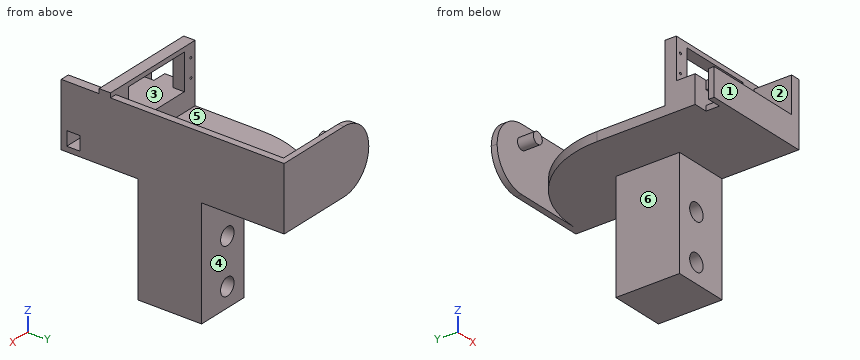
```python
from build123d import *

# Parameters (mm, degrees)
SKETCH1_W            = 55.49400001
SKETCH1_H            = 26.874
BOSS_EXTRUDE1_DEPTH  = 6.35
SKETCH2_W            = 40
SKETCH2_H            = 19
CUT_EXTRUDE1_DEPTH   = 6.35
SKETCH3_R            = 0.635
CUT_EXTRUDE2_DEPTH   = 6.35
SKETCH4_W            = 55.49400001
SKETCH4_H            = 7.874
BOSS_EXTRUDE2_DEPTH  = 21.15
SKETCH6_W            = 7.747000005
SKETCH6_H            = 6.35
BOSS_EXTRUDE3_DEPTH  = 1
SKETCH12_W           = 7.747000005
SKETCH12_H           = 7.475
CUT_EXTRUDE4_DEPTH   = 9.398
SKETCH13_W           = 7.747000005
SKETCH13_H           = 7.9
BOSS_EXTRUDE6_DEPTH  = 20
SKETCH14_W           = 27.874
SKETCH14_H           = 27.5
BOSS_EXTRUDE7_DEPTH  = 5.08
SKETCH16_W           = 3.81
SKETCH16_H           = 27.874
BOSS_EXTRUDE8_DEPTH  = 93.66
BOSS_EXTRUDE9_DEPTH  = 7.62
SKETCH18_W           = 5.08
SKETCH18_H           = 93.66
BOSS_EXTRUDE10_DEPTH = 56.76400001
SKETCH19_W           = 30.48
SKETCH19_H           = 35.56
BOSS_EXTRUDE11_DEPTH = 76.2
SKETCH20_R           = 4.813300002
SKETCH20_R_2         = 4.813299999
CUT_EXTRUDE5_DEPTH   = 76.2
SKETCH21_W           = 30.48
SKETCH21_H           = 35.56
CUT_EXTRUDE6_DEPTH   = 15.24
SKETCH23_W           = 7.876812164
SKETCH23_H           = 7.475
CUT_EXTRUDE7_DEPTH   = 54.102
FILLET1_R            = 55.88
SKETCH24_W           = 3.81
SKETCH24_H           = 35.494
BOSS_EXTRUDE12_DEPTH = 3.302
SKETCH25_W           = 35.494
SKETCH25_H           = 3.302
BOSS_EXTRUDE13_DEPTH = 56.76400001
FILLET2_R            = 17.78
SKETCH26_R           = 3.175
BOSS_EXTRUDE14_DEPTH = 8.89
SKETCH27_W           = 7.747000005
SKETCH27_H           = 20
CUT_EXTRUDE9_DEPTH   = 10.668
SKETCH28_W           = 7.747000005
SKETCH28_H           = 6.35
BOSS_EXTRUDE15_DEPTH = 2.54
SKETCH29_W           = 2.54
SKETCH29_H           = 6.35
BOSS_EXTRUDE16_DEPTH = 47.747000005
SKETCH30_W           = 2.54
SKETCH30_H           = 6.35
BOSS_EXTRUDE17_DEPTH = 5.08


with BuildPart() as part:
    # Sketch1 → Boss-Extrude1 (new body)
    with BuildSketch(Plane(origin=(0, 0, 0), x_dir=(1, 0, 0), z_dir=(0, 1, 0))):
        with Locations((27.747000005, 13.437)):
            Rectangle(SKETCH1_W, SKETCH1_H)
    extrude(amount=BOSS_EXTRUDE1_DEPTH)

    # Sketch2 → Cut-Extrude1 (cut)
    with BuildSketch(Plane(origin=(0, 6.35, 0), x_dir=(1, 0, 0), z_dir=(0, 1, 0))):
        with Locations((27.747000005, 9.5)):
            Rectangle(SKETCH2_W, SKETCH2_H)
    extrude(amount=-CUT_EXTRUDE1_DEPTH, mode=Mode.SUBTRACT)

    # Sketch3 → Cut-Extrude2 (cut)
    with BuildSketch(Plane.XZ):
        with Locations(Location((2.997000004, -14.099999999, 0), (0, 0, 270))):
            Circle(SKETCH3_R)
        with Locations(Location((2.997000004, -3.899999999, 0), (0, 0, 270))):
            Circle(SKETCH3_R)
        with Locations(Location((52.497000004, -14.099999999, 0), (0, 0, 270))):
            Circle(SKETCH3_R)
        with Locations(Location((52.497000004, -3.899999999, 0), (0, 0, 270))):
            Circle(SKETCH3_R)
    extrude(amount=-CUT_EXTRUDE2_DEPTH, mode=Mode.SUBTRACT)

    # Sketch4 → Boss-Extrude2 (add)
    with BuildSketch(Plane.XZ):
        with Locations((27.747000005, -22.937)):
            Rectangle(SKETCH4_W, SKETCH4_H)
    extrude(amount=BOSS_EXTRUDE2_DEPTH)

    # Sketch6 → Boss-Extrude3 (add)
    with BuildSketch(Plane.XY):
        with Locations((3.873500003, 3.175)):
            Rectangle(SKETCH6_W, SKETCH6_H)
        with Locations((51.620500007, 3.175)):
            Rectangle(SKETCH6_W, SKETCH6_H)
    extrude(amount=BOSS_EXTRUDE3_DEPTH)

    # Sketch12 → Cut-Extrude4 (cut)
    with BuildSketch(Plane.XY.offset(-19)):
        with Locations((3.873500003, -14.3125)):
            Rectangle(SKETCH12_W, SKETCH12_H)
    extrude(amount=-CUT_EXTRUDE4_DEPTH, mode=Mode.SUBTRACT)

    # Sketch13 → Boss-Extrude6 (add)
    with BuildSketch(Plane.XY.offset(-19)):
        with Locations((51.620500007, -17.2)):
            Rectangle(SKETCH13_W, SKETCH13_H)
    extrude(amount=BOSS_EXTRUDE6_DEPTH)

    # Sketch14 → Boss-Extrude7 (add)
    with BuildSketch(Plane(origin=(55.49400001, 0, 0), x_dir=(0, 0, -1), z_dir=(1, 0, 0))):
        with Locations((12.937, -7.4)):
            Rectangle(SKETCH14_W, SKETCH14_H)
    extrude(amount=BOSS_EXTRUDE7_DEPTH)

    # Sketch16 → Boss-Extrude8 (add)
    with BuildSketch(Plane(origin=(0, 6.35, 0), x_dir=(1, 0, 0), z_dir=(0, 1, 0))):
        with Locations((58.66900001, 12.937)):
            Rectangle(SKETCH16_W, SKETCH16_H)
    extrude(amount=BOSS_EXTRUDE8_DEPTH)

    # Sketch17 → Boss-Extrude9 (add)
    with BuildSketch(Plane(origin=(0, 0, -26.874), x_dir=(-1, 0, 0), z_dir=(0, 0, -1))):
        Polygon((0, -21.15), (0, -18.05), (-7.747000005, -18.05), (-7.747000005, -10.575), (0, -10.575), (0, 6.35), (-56.76400001, 6.35), (-56.76400001, 100.01), (-60.57400001, 100.01), (-60.57400001, -21.15), align=None)
    extrude(amount=BOSS_EXTRUDE9_DEPTH)

    # Sketch18 → Boss-Extrude10 (add)
    with BuildSketch(Plane.ZY.offset(-56.76400001)):
        with Locations((-31.954, 53.18)):
            Rectangle(SKETCH18_W, SKETCH18_H)
    extrude(amount=BOSS_EXTRUDE10_DEPTH)

    # Sketch19 → Boss-Extrude11 (add)
    with BuildSketch(Plane(origin=(0, 0, -34.494), x_dir=(-1, 0, 0), z_dir=(0, 0, -1))):
        with Locations((-45.33400001, 39.43)):
            Rectangle(SKETCH19_W, SKETCH19_H)
    extrude(amount=BOSS_EXTRUDE11_DEPTH)

    # Sketch20 → Cut-Extrude5 (cut)
    with BuildSketch(Plane.XZ.offset(-21.65)):
        with Locations((42.150157054, -59.253068288)):
            Circle(SKETCH20_R)
        with Locations((42.150157054, -84.653068288)):
            Circle(SKETCH20_R_2)
    extrude(amount=-CUT_EXTRUDE5_DEPTH, mode=Mode.SUBTRACT)

    # Sketch21 → Cut-Extrude6 (cut)
    with BuildSketch(Plane(origin=(0, 0, -110.694), x_dir=(-1, 0, 0), z_dir=(0, 0, -1))):
        with Locations((-45.33400001, 39.43)):
            Rectangle(SKETCH21_W, SKETCH21_H)
    extrude(amount=-CUT_EXTRUDE6_DEPTH, mode=Mode.SUBTRACT)

    # Sketch23 → Cut-Extrude7 (cut)
    with BuildSketch(Plane.ZY.offset(-7.747000005)):
        with Locations((-27.675104405, -14.3125)):
            Rectangle(SKETCH23_W, SKETCH23_H)
    extrude(amount=-CUT_EXTRUDE7_DEPTH, mode=Mode.SUBTRACT)

    # Fillet1
    fillet1_edges = [part.edges().sort_by_distance(p)[0] for p in [
        (0, 100.01, -31.954),
    ]]
    fillet(fillet1_edges, radius=FILLET1_R)

    # Sketch24 → Boss-Extrude12 (add)
    with BuildSketch(Plane(origin=(0, 100.01, 0), x_dir=(1, 0, 0), z_dir=(0, 1, 0))):
        with Locations((58.66900001, 16.747)):
            Rectangle(SKETCH24_W, SKETCH24_H)
    extrude(amount=BOSS_EXTRUDE12_DEPTH)

    # Sketch25 → Boss-Extrude13 (add)
    with BuildSketch(Plane.ZY.offset(-56.76400001)):
        with Locations((-16.747, 101.661)):
            Rectangle(SKETCH25_W, SKETCH25_H)
    extrude(amount=BOSS_EXTRUDE13_DEPTH)

    # Fillet2
    # the kernel refuses this fillet: 17.78 mm, written as the material it takes off along each edge
    with BuildSketch(Plane(origin=(0, 55.56, 1), x_dir=(0, 0, -1), z_dir=(0, 1, 0))) as fillet2_piece_1:
        with BuildLine():
            CenterArc((FILLET2_R, -FILLET2_R), FILLET2_R, 90, 90)
            Line((0, -FILLET2_R), (0, 0))
            Line((0, 0), (FILLET2_R, 0))
        make_face()
    extrude(amount=92.202000001, mode=Mode.SUBTRACT)
    with BuildSketch(Plane(origin=(0, 147.762, -34.494), x_dir=(0, 0, 1), z_dir=(0, -1, 0))) as fillet2_piece_2:
        with BuildLine():
            CenterArc((FILLET2_R, -FILLET2_R), FILLET2_R, 90, 90)
            Line((0, -FILLET2_R), (0, 0))
            Line((0, 0), (FILLET2_R, 0))
        make_face()
    extrude(amount=47.752, mode=Mode.SUBTRACT)

    # Sketch26 → Boss-Extrude14 (add)
    with BuildSketch(Plane(origin=(0, 100.01, 0), x_dir=(1, 0, 0), z_dir=(0, 1, 0))):
        with Locations(Location((17.747000004, 8.999999999, 0), (0, 0, 270))):
            Circle(SKETCH26_R)
    extrude(amount=-BOSS_EXTRUDE14_DEPTH)

    # Sketch27 → Cut-Extrude9 (cut)
    with BuildSketch(Plane.XZ.offset(21.15)):
        with Locations((51.620500007, -9)):
            Rectangle(SKETCH27_W, SKETCH27_H)
    extrude(amount=-CUT_EXTRUDE9_DEPTH, mode=Mode.SUBTRACT)

    # Sketch28 → Boss-Extrude15 (add)
    with BuildSketch(Plane.XY.offset(1)):
        with Locations((51.620500007, 3.175)):
            Rectangle(SKETCH28_W, SKETCH28_H)
    extrude(amount=BOSS_EXTRUDE15_DEPTH)

    # Sketch29 → Boss-Extrude16 (add)
    with BuildSketch(Plane.ZY.offset(-47.747000005)):
        with Locations((2.27, 3.175)):
            Rectangle(SKETCH29_W, SKETCH29_H)
    extrude(amount=BOSS_EXTRUDE16_DEPTH)

    # Sketch30 → Boss-Extrude17 (add)
    with BuildSketch(Plane(origin=(55.49400001, 0, 0), x_dir=(0, 0, -1), z_dir=(1, 0, 0))):
        with Locations((-2.27, 3.175)):
            Rectangle(SKETCH30_W, SKETCH30_H)
    extrude(amount=BOSS_EXTRUDE17_DEPTH)


solid = part.part
```
Verification items for the finished model (mm, model axes). Face numbers are marked on the shaded views. A direction names the side the tool comes from. Give positions to 0.01 mm unless a question says otherwise; leave off trailing zeros. Order: outer loops, then holes, each group sorted by start corner. A loop starts at its lowest first (then second) coordinate and runs counter-clockwise, first axis right, second up. Notation, with made-up numbers: M 63.25,60 L 100.25,60 A21 cw 100.25,93 Z; hole C 24,-21.75 d6. An arc over 180 degrees is marked long. Return JSON: item names as keys, results as strings. Group by question number.
1) Section check B-B on z = -10. Record the cut outline in (x, y), and give its area (3 significant figures).
2) Section check C-C on y = -7. Record the cut outline in (x, z).
3) Section check D-D on y = 18. Record the cut outline in (x, z).
4) Mould release check, pull along X, two halves, no side actions. Record for the marked faces 1, 2 and 3: pulls with the +X half, pulls with the -X half, needs draft (parallel to the pull), parting line crosses it, or undercut.
5) Scan lines: line 1 (X direction, y = 2.25, z = -14.1); line 2 (Z direction, x = 51.5, y = -15); line 3 (Y direction, x = 20, z = -24) (3 decimals). Record each from-to range of solid material in increasing order.
6) Access from +Z, -Z, +X, -X, +Y, -Y to the whole of each face (thin tool, end or side, straight path). Record for the marked faces 4, 5 and 6.
7) Go/stop test with flat-tipped pins: pin 1 Ø6 at (x, y) = (38.5, 16.5) entering from -Z; pin 2 Ø2 at (x, y) = (39, -13.5) entering from +Z; pin 3 Ø2 at (x, y) = (49.5, 27) entering from +Z; pin 4 Ø7.5 at (x, z) = (42.15, -84.65) entering from +Y. Record where each tip stops, or that it passes through.
8) Section check A-A on x = 43. Give the number of separate pieces and of enclosed holes in the cut face, and give its area (3 significant figures).
Answer block:
{
 "1": {"outline": "M 0,0 L 7.75,0 L 7.75,6.35 L 0,6.35 Z; M 1.34,100.01 L 14.73,100.01 L 14.73,91.12 L 20.76,91.12 L 20.76,100.01 L 56.76,100.01 L 56.76,6.35 L 47.75,6.35 L 47.75,0 L 55.49,0 L 55.49,-21.15 L 60.57,-21.15 L 60.57,103.31 L 1.34,103.31 Z", "area": "844 mm^2"},
 "2": {"outline": "M 0,-34.49 L 60.57,-34.49 L 60.57,1 L 55.49,1 L 55.49,-19 L 0,-19 Z"},
 "3": {"outline": "M 0,-34.49 L 60.57,-34.49 L 60.57,1 L 56.76,1 L 56.76,-29.41 L 0,-29.41 Z"},
 "4": {"face 1": "needs draft", "face 2": "pulls with the -X half", "face 3": "undercut"},
 "5": {"line 1": "x = 0 to 2.36, 3.63 to 7.75, 47.75 to 51.86, 53.13 to 60.57", "line 2": "z = -34.49 to -31.61, -23.74 to -19", "line 3": "y = -21.15 to -18.05, -10.575 to 6.35, 100.01 to 103.312"},
 "6": {"face 4": "-Z, +X, -X, +Y", "face 5": "+Z, -X", "face 6": "-Z, -X, +Y, -Y"},
 "7": {"pin 1": "stops at z = -34.49", "pin 2": "stops at z = -19", "pin 3": "stops at z = -29.41", "pin 4": "passes through"},
 "8": {"separate pieces": "5", "enclosed holes": "1", "area": "2,460 mm^2"}
}
